Job drawing, mm, ordinate dimensions from the low corner. One solid piece. Coordinates: 2 decimals unless noted, no trailing zeros. Order: outer loops, then holes, each group sorted by start corner. A loop starts at its lowest first (then second) coordinate and runs counter-clockwise, first axis right, second up. Notation, with made-up numbers: (15, 1.25) - (45, 1.25) arc R10 ccw to (45, 19.25) - close; hole circle Ø1 at (-23, 10.5). An arc over 180 degrees is marked (long way). Return JSON: item names as keys, results as strings.
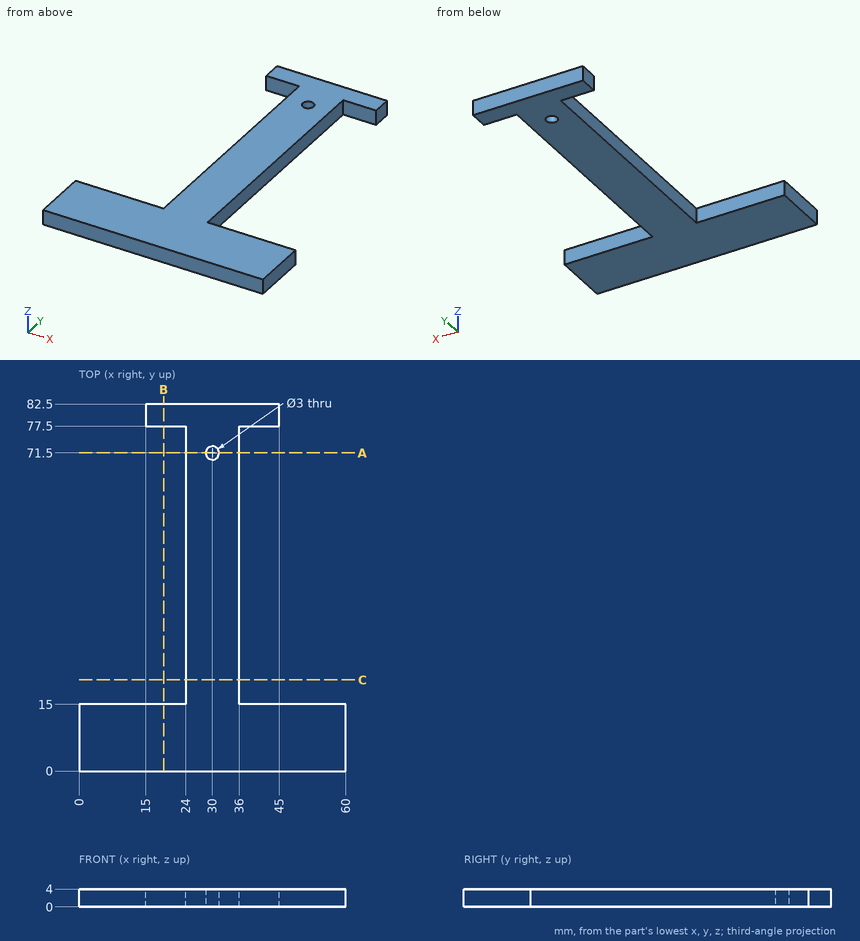
1. Drop flat-ended pins along their axis: pin 1 (1.2 mm diameter, centred on x = 11.5, z = 1.5, fed in from +Y); pin 2 (1.2 mm diameter, centred on y = 42, z = 3, fed in from -X). Give the stop position or say it passes through.
Check values:
{"pin 1": "y = 15", "pin 2": "x = 24"}
2. Cut at A-A on y = 71.5. Give the cut face in (x, z), plus the area to 3 significant figures.
Check values:
{"outline": "(24, 0) - (28.5, 0) - (28.5, 4) - (24, 4) - close; (31.5, 0) - (36, 0) - (36, 4) - (31.5, 4) - close", "area": "36.0 mm²"}
3. Cut at B-B on x = 19. Give the cut face in (y, z), plus the area to 3 significant figures.
Check values:
{"outline": "(0, 0) - (15, 0) - (15, 4) - (0, 4) - close; (77.5, 0) - (82.5, 0) - (82.5, 4) - (77.5, 4) - close", "area": "80.0 mm²"}
4. Cut at C-C on y = 20.5. Give the cut face in (x, z), plus the area to 3 significant figures.
Check values:
{"outline": "(24, 0) - (36, 0) - (36, 4) - (24, 4) - close", "area": "48.0 mm²"}
5. Probe L1, parallel to Y at x = 43, z = 3.65; L2, parallel to X at y = 71.5, z = 2.4; L3, parallel to Y at x = 30, z = 1.3. List the from-to ranges inside material, lowest first.
Check values:
{"L1": "0 to 15, 77.5 to 82.5", "L2": "24 to 28.5, 31.5 to 36", "L3": "0 to 70, 73 to 82.5"}
